Check sheet for the modelled part. Datum: model origin and axes. Units: mm. A direction names the side the tool comes from. Give positions to 0.01 mm unless a question says otherwise; leave off trailing zeros. Write each loop counter-clockwise with the first axis right and the second up, starting at its lowest first coordinate (ties: lowest second). Pieces come first, ordered by that corner, then holes. Notation, with made-up numbers: M 37,27 L 44,27 A29 ccw 44,49 Z; hole C -21.75,52.5 d11. An arc over 180 degrees is marked long. Write item = value, one per line. Start each with the question number.
1) Set-up check for faces 4 (the face through (1, -3.8, 2)), 5 (the face through (3.3, 0, 4)), 6 (the face through (-0.1, 3.5, 2)), 7 (the face through (-3.8, 0, 4)), 8 (the face through (-1, 3.8, 2)): record each of +Z, -Z, +X, -X, +Y, -Y from which the full face is reachable in a straight line by a thin tool's end or side.
2) Draft check along X on faces 1 (the face through (1, 3.3, 2)), 2 (the face through (0, 0, 0)), 3 (the face through (3.8, 0, 4)). Enter one of: pulls with the +X half, pulls with the -X half, needs draft (parallel to the pull), parting line crosses it, or undercut.
3) Scan lines: L1, parallel to X at y = -1, z = 5.5; L2, parallel to Z at x = 0.5, y = -1.5. Record each from-to range of solid material in increasing order.
4) Sectioned sample at A-A, the plane z = 5.5. Record the cut outline in (x, y).
5) Sectioned sample at B-B, the plane x = -3. Record the cut outline in (y, z).
6) Gauge pin test, flat ends, axial feed: pin 1 (0.6 mm diameter, centred on y = -3.5, z = 5.5, fed in from +X); pin 2 (3 mm diameter, centred on y = 1, z = 5.5, fed in from -X); pin 3 (1 mm diameter, centred on x = -1.5, y = 1, fed in from +Z); pin 4 (5.5 mm diameter, centred on x = -0.5, y = 1.5, fed in from +Z). Record the tip position at first contact, or that the pin passes through.
7) Sectioned sample at C-C, the plane z = 1.25. Record the cut outline in (x, y).
Solid Edge part; units mm, degrees
sketch "Sketch1" plane through (0, 0, 0) normal (0, 0, 1) x (1, 0, 0)
  line L0 (5, -5) -> (5, 5)
  line L1 (5, 5) -> (-5, 5)
  line L2 (-5, 5) -> (-5, -5)
  line L3 (-5, -5) -> (5, -5)
extrude "Protrusion1" add sketch "Sketch1" along normal blind 1
sketch "Sketch2" plane through (0, 0, 1) normal (0, 0, 1) x (1, 0, 0)
  line L0 (-3.3, -3.3) -> (3.3, -3.3)
  line L1 (3.3, -3.3) -> (3.3, 3.3)
  line L2 (3.3, 3.3) -> (-3.3, 3.3)
  line L3 (-3.3, 3.3) -> (-3.3, -3.3)
  line L4 (3.8, -3.8) -> (-3.8, -3.8)
  line L5 (-3.8, -3.8) -> (-3.8, 3.8)
  line L6 (-3.8, 3.8) -> (3.8, 3.8)
  line L7 (3.8, 3.8) -> (3.8, -3.8)
extrude "ExtrudedProtrusion_2" add sketch "Sketch2" along normal blind 7
sketch "Sketch3" plane through (0, -3.8, 4.5) normal (0, -1, 0) x (1, 0, 0)
  line L0 (2.5, 3.5) -> (2.5, 0)
  arc A0 (-2.5, 0) -> (2.5, 0) centre (0, 0) ccw
  line L1 (-2.5, 0) -> (-2.5, 3.5)
  line L2 (-2.5, 3.5) -> (2.5, 3.5)
extrude "ExtrudedCutout_1" cut sketch "Sketch3" against normal blind 9.3
fillet "Round_1" radius 0.5 4 edges at (0, -5, 0) (5, 0, 0) (0, 5, 0) (-5, 0, 0)
properties material "ABS Plastic, high impact"
Data:
q1.face_4 = +Z, +X, -X, -Y
q1.face_5 = +Z
q1.face_6 = +Z, +Y, -Y
q1.face_7 = +Z, -X, +Y, -Y
q1.face_8 = +Z, +X, -X, +Y
q2.face_1 = undercut
q2.face_2 = needs draft
q2.face_3 = pulls with the +X half
q3.L1 = -3.8 to -3.3, 3.3 to 3.8
q3.L2 = 0 to 1
q4.outline = M -3.8,-3.8 L -2.5,-3.8 L -2.5,-3.3 L -3.3,-3.3 L -3.3,3.3 L -2.5,3.3 L -2.5,3.8 L -3.8,3.8 Z; M 2.5,-3.8 L 3.8,-3.8 L 3.8,3.8 L 2.5,3.8 L 2.5,3.3 L 3.3,3.3 L 3.3,-3.3 L 2.5,-3.3 Z
q5.outline = M -5,0.5 A0.5 ccw -4.5,0 L 4.5,0 A0.5 ccw 5,0.5 L 5,1 L 3.8,1 L 3.8,8 L 3.3,8 L 3.3,1 L -3.3,1 L -3.3,8 L -3.8,8 L -3.8,1 L -5,1 Z
q6.pin_1 = 3.8
q6.pin_2 = -3.8
q6.pin_3 = 1
q6.pin_4 = 8
q7.outline = M -3.8,-3.8 L 3.8,-3.8 L 3.8,3.8 L -3.8,3.8 Z; hole M -3.3,-3.3 L 3.3,-3.3 L 3.3,3.3 L -3.3,3.3 Z
